Input: dimensioned drawing with shaded views. Units: mm. Origin: part minimum x, y, z. Coordinates: 2 decimals unless noted, no trailing zeros. Write each loop counter-clockwise with the first axis right and the second up, starting at its lowest first coordinate (ties: lowest second). Pieces come first, ordered by that corner, then holes. Notation, with made-up numbers: M -35,60.25 L -6,60.25 A17 cw -6,76.25 Z; hole C 1.25,-13 d4. An arc over 180 degrees is marked long. Use one line per item in the form item = value.
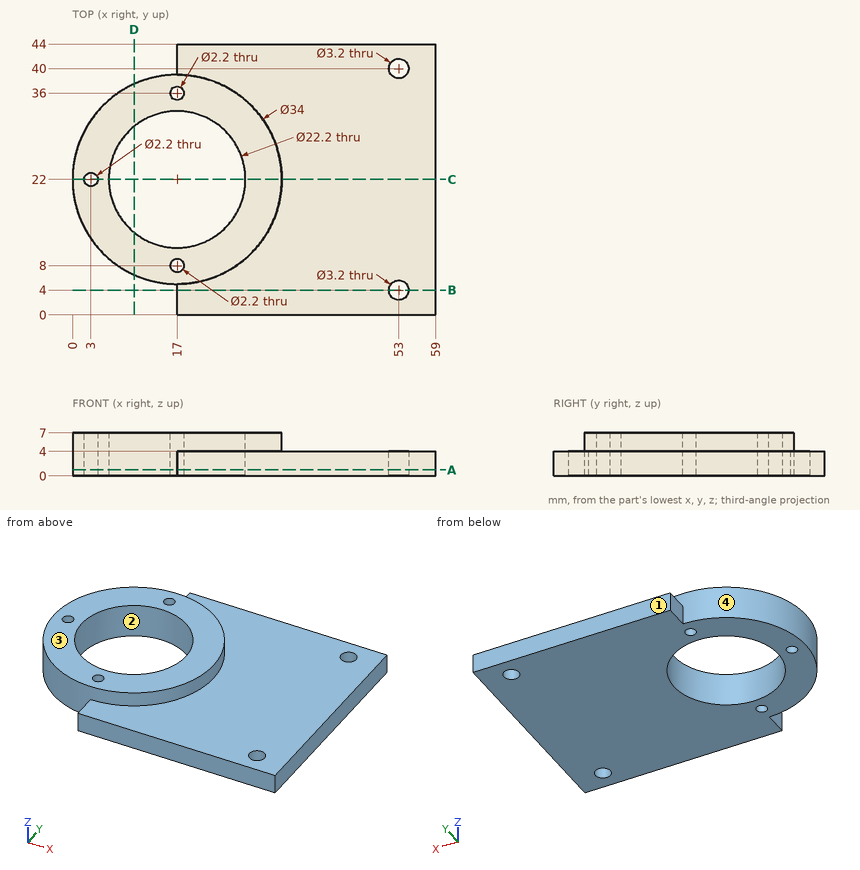
(1) Section query C-C on y = 22. Return the cut outline in (x, z), plus the area to 3 significant figures.
Computed:
outline = M 0,0 L 1.9,0 L 1.9,7 L 0,7 Z; M 4.1,0 L 5.9,0 L 5.9,7 L 4.1,7 Z; M 28.1,0 L 59,0 L 59,4 L 34,4 L 34,7 L 28.1,7 Z
area = 167 mm^2
(2) Section query A-A on z = 1. Return the cut outline in (x, y), plus the area to 3 significant figures.
Computed:
outline = M 17,0 L 59,0 L 59,44 L 17,44 L 17,39 A17 ccw 17,5 Z; hole C 3,22 d2.2; hole C 17,22 d22.2; hole C 17,8 d2.2; hole C 17,36 d2.2; hole C 53,4 d3.2; hole C 53,40 d3.2
area = 1,890 mm^2
(3) Section query D-D on x = 10. Return the cut outline in (y, z), plus the area to 3 significant figures.
Computed:
outline = M 6.51,0 L 13.39,0 L 13.39,7 L 6.51,7 Z; M 30.61,0 L 37.49,0 L 37.49,7 L 30.61,7 Z
area = 96.3 mm^2
(4) Line query: probe 1 along Y at (x, z) = (53, 3.1); probe 2 along X at (y, z) = (15.5, 2.5); probe 3 along Z at (x, y) = (48.5, 37). Output: solid intervals per line, ascending.
Computed:
probe_1 = 0 to 2.4, 5.6 to 38.4, 41.6 to 44
probe_2 = 1.29 to 8, 26 to 59
probe_3 = 0 to 4
(5) Pull-direction query (Y, two-part tool) for the marked faces 1, 2, 3 and 4; classes: pulls with the +Y half, pulls with the -Y half, needs draft (parallel to the pull), parting line crosses it, or undercut.
Computed:
face_1 = pulls with the +Y half
face_2 = undercut
face_3 = needs draft
face_4 = parting line crosses it
(6) Section query B-B on y = 4. Return the cut outline in (x, z).
Computed:
outline = M 17,0 L 51.4,0 L 51.4,4 L 17,4 Z; M 54.6,0 L 59,0 L 59,4 L 54.6,4 Z
(7) First-contact query: pin 1 Ø4 at (x, y) = (52.5, 37) entering from +Z; pin 2 Ø1.2 at (y, z) = (3, 1.5) entering from -X. Flat tips, straight axial feed; report the tip coordinate or a pass-through.
Computed:
pin_1 = 4
pin_2 = 17
